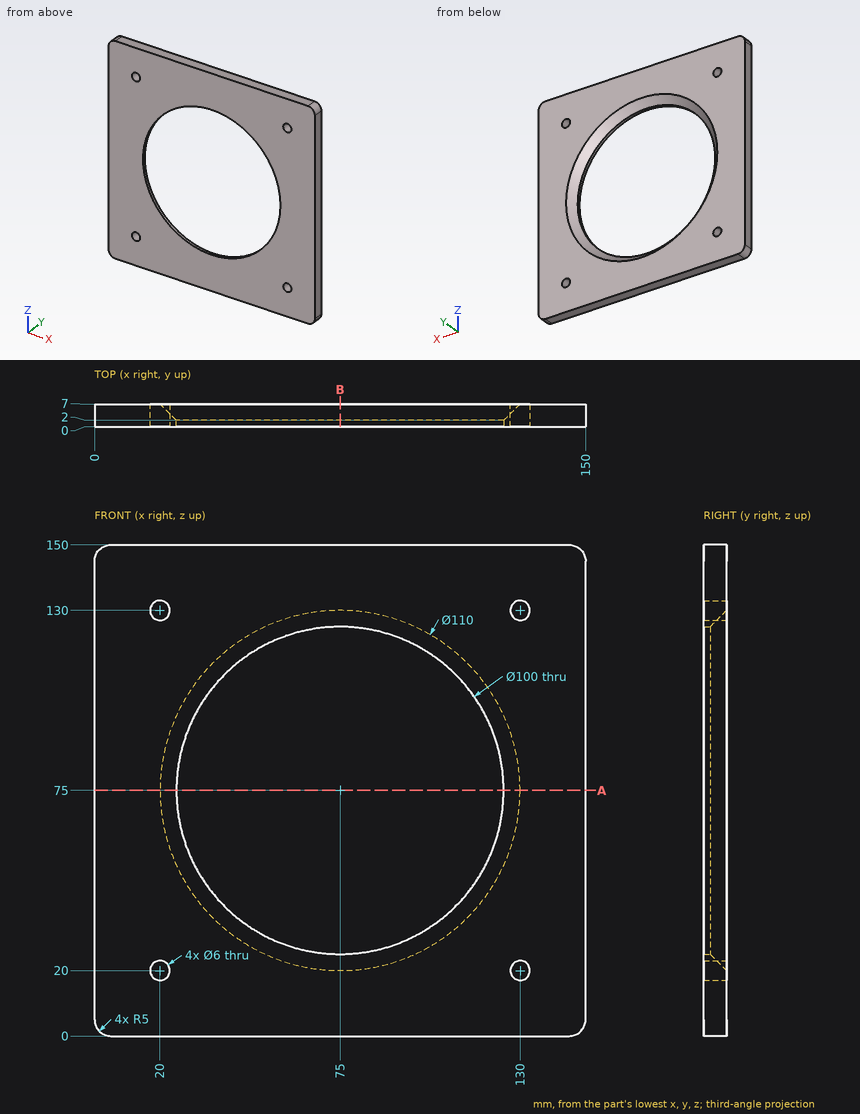
Study the drawing (mm; zero at the part's minimum x, y, z) and answer. Give positions to 0.01 mm unless a question says otherwise; leave off trailing zeros. Loops run counter-clockwise (first coordinate to the right, second up) from the corner with the lowest first, then second, coordinate; pieces in that order, holes last. Notation, with made-up numbers: (-38.5, 11.25) - (-25.5, 11.25) arc R22 ccw to (-25.5, 27.25) - close; hole circle Ø8 at (-24, 62). An arc over 180 degrees is marked (long way). One line per question, with ' | ' between items.
(1) The part is cut by section B-B (x = 75). Write down the section's boundary in (y, z), then the cut area to 3 significant figures.
Recorded:
outline: (0, 0) - (7, 0) - (7, 20) - (2, 25) - (0, 25) - close; (0, 125) - (2, 125) - (7, 130) - (7, 150) - (0, 150) - close | area: 325 mm²
(2) The part is cut by section A-A (z = 75). Write down the section's boundary in (x, y).
Recorded:
outline: (0, 0) - (25, 0) - (25, 2) - (20, 7) - (0, 7) - close; (125, 0) - (150, 0) - (150, 7) - (130, 7) - (125, 2) - close
(3) Straight lines are drawn through the part: probe 1 along Z at (x, y) = (130, 3.25); probe 2 along Z at (x, y) = (77, 1.75). For each, find the intervals that lie inside material, in ascending order.
Recorded:
probe 1: z = 0 to 17, 23 to 127, 133 to 150 | probe 2: z = 0 to 25.04, 124.96 to 150
